Could you check a few things on this model? Use its own coordinates, in mm. Face numbers are marked on the shaded views. A direction names the side the tool comes from. Coordinates: 2 decimals unless noted, no trailing zeros. Write each loop counter-clockwise with the first axis right and the second up, starting at its lowest first coordinate (ties: lowest second). Pieces come first, ordered by that corner, then holes. Notation, with made-up numbers: M -39,-10 L 2,-10 A9 cw 2,4 Z; hole C 56.5,-3.75 d10. An arc over 180 degrees is marked long. Answer as CSV lines item,"result". Start each with the question number.
Item 1: We'd pull the mould along X, two halves only. Please class the marked faces 3, 4, 5 and 6: +X half, -X half, draft (parallel to the pull), parting line (faces both ways), or undercut.
Item 2: If I drill on line 1 along Z through (x, y) = (0, -12.5) (3 decimals); line 2 along X through (y, z) = (-17.75, 123.5); line 3 along Z through (x, y) = (-12.5, -23.75), over which ranges is the centre line in solid material (lowest first)? Write a range as [from, to].
Item 3: On a 3-axis mill with a long thin cutter (end or side, diameter ignored), from which of +Z, -Z, +X, -X, +Y, -Y can I reach the whole of each face in a straight line? I mean the marked faces 1 and 2. Say none if no direction works.
Item 4: Suppose I cut it at B-B, the plane x = -4. Write out the boundary of the cut face in (y, z).
Item 5: I'm going to push flat-ended pins straight in: P1, Ø5, axis at y = -21, z = 41.5, coming from the +X side; P2, Ø6, axis at y = -10, z = 84, coming from the -X side; P3, Ø2, axis at y = -8, z = 98.5, coming from the -X side. Where does each tip first touch, or does it pass through?
Item 6: Suppose I cut it at D-D, the plane x = 76.2. Write out the boundary of the cut face in (y, z).
Item 7: Suppose I cut it at A-A, the plane z = 61. Write out the boundary of the cut face in (x, y).
Item 8: Suppose I cut it at C-C, the plane y = -20.75. State how many separate pieces and enclosed holes the cut face has, and give its area (3 significant figures).
```python
from build123d import *

# Parameters (mm, degrees)
F0_R     = 12.7
F1_DEPTH = 25.4


with BuildPart() as f1:
    # F0 (on Front) → F1 (new body)
    with BuildSketch(Plane.XZ):
        with BuildLine():
            ThreePointArc((-105.440213, 76.098159), (-54.724054, 56.469184), (-37.797935, 4.788124))
            ThreePointArc((-37.797935, 4.788124), (-28.58354, -25.191095), (0, -38.1))
            ThreePointArc((0, -38.1), (19.733421, -32.591442), (33.760663, -17.658641))
            Line((33.760663, -17.658641), (104.333886, 117.266737))
            ThreePointArc((104.333886, 117.266737), (106.690251, 140.83705), (92.075, 159.478578))
            ThreePointArc((92.075, 159.478578), (-24.036398, 182.574571), (-130.213714, 130.213714))
            ThreePointArc((-130.213714, 130.213714), (-139.513073, 107.763073), (-130.213714, 85.312433))
            ThreePointArc((-130.213714, 85.312433), (-118.831388, 78.004799), (-105.440213, 76.098159))
        make_face()
        with BuildLine():
            ThreePointArc((0, 15.875), (11.22532, 11.22532), (15.875, 0))
            ThreePointArc((15.875, 0), (-11.22532, -11.22532), (0, 15.875))
        make_face(mode=Mode.SUBTRACT)
        with Locations((-107.763073, 107.763073)):
            Circle(F0_R, mode=Mode.SUBTRACT)
        with BuildLine():
            ThreePointArc((17.011753, 30.501736), (8.760735, 33.448122), (0, 33.548198))
            ThreePointArc((0, 33.548198), (-9.556693, 35.925334), (-14.541131, 44.418657))
            ThreePointArc((-14.541131, 44.418657), (-41.266263, 81.937069), (-83.376373, 100.607971))
            ThreePointArc((-83.376373, 100.607971), (-88.168492, 105.162713), (-89.886657, 111.546911))
            ThreePointArc((-89.886657, 111.546911), (-89.905581, 121.02761), (-90.171772, 130.50459))
            ThreePointArc((-90.171772, 130.50459), (-86.184302, 141.607355), (-75.583098, 146.782851))
            ThreePointArc((-75.583098, 146.782851), (-17.617296, 164.157366), (42.715256, 159.478578))
            ThreePointArc((42.715256, 159.478578), (48.987823, 153.432961), (47.199631, 144.906711))
            ThreePointArc((47.199631, 144.906711), (46.002172, 122.176475), (60.325, 104.485965))
            ThreePointArc((60.325, 104.485965), (67.14271, 95.600952), (65.680907, 84.49745))
            Line((65.680907, 84.49745), (37.821481, 36.243509))
            ThreePointArc((37.821481, 36.243509), (28.593318, 29.107942), (17.011753, 30.501736))
        make_face(mode=Mode.SUBTRACT)
        with Locations((76.2, 131.982272)):
            Circle(F0_R, mode=Mode.SUBTRACT)
    extrude(amount=F1_DEPTH)


solid = f1.part
```
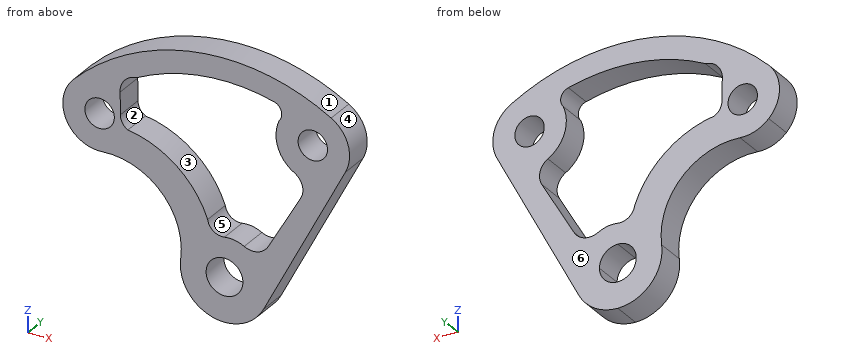
Ans:
1,face 3,"undercut"
1,face 4,"+X half"
1,face 5,"undercut"
1,face 6,"draft"
2,line 1,"z = [-38.1, -15.875], [15.875, 33.548], [165.1, 184.15]"
2,line 2,"x = [-135.34, -89.95], [45.6, 66.75], [85.65, 106.8]"
2,line 3,"z = [-35.99, -9.79], [9.79, 39.02], [164.63, 183.73]"
3,face 1,"+Z, +Y, -Y"
3,face 2,"+Y, -Y"
4,outline,"M -25.4,-37.89 L 0,-37.89 L 0,-15.36 L -25.4,-15.36 Z; M -25.4,15.36 L 0,15.36 L 0,33.56 L -25.4,33.56 Z; M -25.4,165.05 L 0,165.05 L 0,184.11 L -25.4,184.11 Z"
5,P1,"stops at x = 66.01"
5,P2,"stops at x = -131.78"
5,P3,"stops at x = -138.42"
6,outline,"M -25.4,63.48 L 0,63.48 L 0,119.28 L -25.4,119.28 Z; M -25.4,144.68 L 0,144.68 L 0,167.64 L -25.4,167.64 Z"
7,outline,"M -59.49,-25.4 L -22.71,-25.4 L -22.71,0 L -59.49,0 Z; M 52.11,-25.4 L 74.9,-25.4 L 74.9,0 L 52.11,0 Z"
8,separate pieces,"1"
8,enclosed holes,"4"
8,area,"16,900 mm^2"
